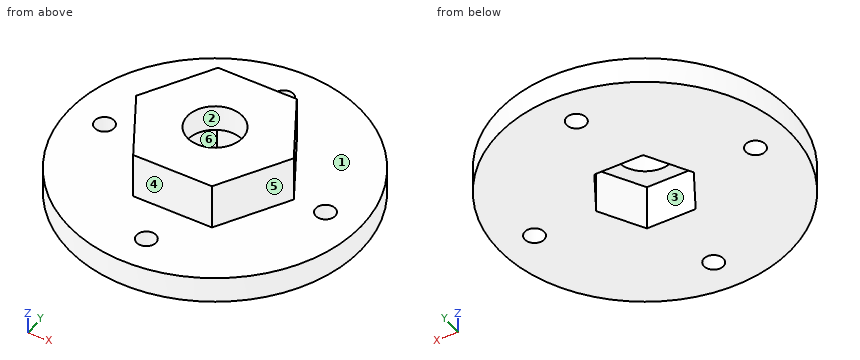
```python
from build123d import *

# Parameters (mm, degrees)
F0_R     = 22.5
F0_R_2   = 1.5
F0_R_3   = 3.75
F1_DEPTH = 4
F0_R_4   = 4.25
F2_DEPTH = 11
F3_DEPTH = 25
F4_DEPTH = 7


with BuildPart() as f1:
    # F0 (on Top) → F1 (new body)
    with BuildSketch(Plane.XY):
        Circle(F0_R)
        with Locations((0, -17)):
            Circle(F0_R_2, mode=Mode.SUBTRACT)
        with Locations((-17, 0)):
            Circle(F0_R_3, mode=Mode.SUBTRACT)
        Polygon((6.062178, -10.5), (-6.062178, -10.5), (-12.124356, 0), (-6.062178, 10.5), (6.062178, 10.5), (12.124356, 0), align=None, mode=Mode.SUBTRACT)
        with Locations((17, 0)):
            Circle(F0_R_2, mode=Mode.SUBTRACT)
        with Locations((0, 17)):
            Circle(F0_R_2, mode=Mode.SUBTRACT)
        with Locations((-17, 0)):
            Circle(F0_R_3)
        with Locations((-17, 0)):
            Circle(F0_R_2, mode=Mode.SUBTRACT)
    extrude(amount=F1_DEPTH)

    # F0 (on Top) → F2 (join)
    with BuildSketch(Plane.XY):
        Polygon((-12.124356, 0), (-6.062178, -10.5), (6.062178, -10.5), (12.124356, 0), (6.062178, 10.5), (-6.062178, 10.5), align=None)
        Polygon((7.505553, 0), (3.752777, -6.5), (-3.752777, -6.5), (-7.505553, 0), (-3.752777, 6.5), (3.752777, 6.5), align=None, mode=Mode.SUBTRACT)
        Polygon((-3.752777, -6.5), (3.752777, -6.5), (7.505553, 0), (3.752777, 6.5), (-3.752777, 6.5), (-7.505553, 0), align=None)
        Circle(F0_R_4, mode=Mode.SUBTRACT)
        Circle(F0_R_4)
    extrude(amount=F2_DEPTH)

    # F0 (on Top) → F3 (cut)
    with BuildSketch(Plane.XY):
        Circle(F0_R_4)
    extrude(amount=F3_DEPTH, mode=Mode.SUBTRACT)

    # F0 (on Top) → F4 (cut)
    with BuildSketch(Plane.XY):
        Polygon((-3.752777, -6.5), (3.752777, -6.5), (7.505553, 0), (3.752777, 6.5), (-3.752777, 6.5), (-7.505553, 0), align=None)
        Circle(F0_R_4, mode=Mode.SUBTRACT)
    extrude(amount=F4_DEPTH, mode=Mode.SUBTRACT)


solid = f1.part
```
Geometry: final body of the model. Coordinates: model frame, mm. Face numbers are marked on the shaded views. A direction names the side the tool comes from. Round coordinates to 2 decimals unless told otherwise and drop trailing zeros. Order: outer loops, then holes, each group sorted by start corner. A loop starts at its lowest first (then second) coordinate and runs counter-clockwise, first axis right, second up. Notation, with made-up numbers: (-33, -14) -> (19, -14) arc R18 cw to (19, 1) -> close; hole circle Ø10 at (-9, 74). An arc over 180 degrees is marked (long way). Write each question's results on one line, items separated by ' | '.
Q1. Section query B-B (z = 2.5). Output: boundary loops of the cut face in (x, y), and give its area (3 significant figures).
Response values:
outline: circle Ø45 at (0, 0); hole circle Ø3 at (-17, 0); hole (-7.51, 0) -> (-3.75, -6.5) -> (3.75, -6.5) -> (7.51, 0) -> (3.75, 6.5) -> (-3.75, 6.5) -> close; hole circle Ø3 at (0, -17); hole circle Ø3 at (0, 17); hole circle Ø3 at (17, 0) | area: 1,420 mm²
Q2. Section query C-C (x = 17). Output: boundary loops of the cut face in (y, z), and give its area (3 significant figures).
Response values:
outline: (-14.74, 0) -> (-1.5, 0) -> (-1.5, 4) -> (-14.74, 4) -> close; (1.5, 0) -> (14.74, 0) -> (14.74, 4) -> (1.5, 4) -> close | area: 106 mm²
Q3. Pin query (flat end, axial travel): pin 1 Ø5 at (x, y) = (-17, 0) entering from +Z; pin 2 Ø2.5 at (x, y) = (17, 0) entering from -Z; pin 3 Ø3.5 at (x, z) = (-2, 9) entering from +Y; pin 4 Ø1 at (y, z) = (-14, 2) entering from -X. Return the tip coordinate at first contact, or that it passes through.
Response values:
pin 1: z = 4 | pin 2: through | pin 3: y = 10.5 | pin 4: x = -18
Q4. Section query A-A (z = 5.75). Output: boundary loops of the cut face in (x, y), and give its area (3 significant figures).
Response values:
outline: (-12.12, 0) -> (-6.06, -10.5) -> (6.06, -10.5) -> (12.12, 0) -> (6.06, 10.5) -> (-6.06, 10.5) -> close; hole (-7.51, 0) -> (-3.75, -6.5) -> (3.75, -6.5) -> (7.51, 0) -> (3.75, 6.5) -> (-3.75, 6.5) -> close | area: 236 mm²
Q5. Ray query, line 1 along Y through (x, z) = (0, 1.15); line 2 along Z through (x, y) = (13, -4); line 3 along Y through (x, z) = (5, 5.5). Return the intervals inside material, ascending.
Response values:
line 1: -22.5 to -18.5, -15.5 to -6.5, 6.5 to 15.5, 18.5 to 22.5 | line 2: 0 to 4 | line 3: -10.5 to -4.34, 4.34 to 10.5
Q6. Pull-direction query (X, two-part tool) for the marked faces 4, 5 and 6; classes: released by +X, released by -X, zero draft, split by the parting line, or undercut.
Response values:
face 4: zero draft | face 5: released by +X | face 6: undercut
Q7. Access query for the marked faces 1, 2 and 3. Directions: +Z, -Z, +X, -X, +Y, -Y. A direction counts if a zero-diameter tool reaches every point of the face in a straight line with its end or side. Return the directions, or none.
Response values:
face 1: +Z | face 2: +Z, -Z | face 3: -Z
